```python
from build123d import *

# Parameters (mm, degrees)
F0_W     = 2
F0_H     = 50
F1_DEPTH = 45
F2_R     = 1.99999
F4_DEPTH = 40


# Not quite as in the source:
# - a fillet or chamfer is up to 0.001 mm smaller than in the source, because OpenCascade refuses the exact size


with BuildPart() as f1:
    # F0 (on Front) → F1 (new body)
    with BuildSketch(Plane.XZ):
        with Locations((-1, 25)):
            Rectangle(F0_W, F0_H)
    extrude(amount=F1_DEPTH)

    # F2 (radius 2 in the source; OpenCascade refuses exactly that, so slightly less here)
    f2_edges = [f1.edges().sort_by_distance(p)[0] for p in [
        (0, -22.5, 0),
        (0, -22.5, 50),
    ]]
    fillet(f2_edges, radius=F2_R)

    # F3 (on face) → F4 (cut)
    with BuildSketch(Plane.XZ.offset(45)):
        with BuildLine():
            Line((-2, 49.4142135624), (-2, 46.4142135624))
            ThreePointArc((-2, 46.4142135624), (-0.5, 47.9142135624), (-2, 49.4142135624))
        make_face()
        with BuildLine():
            ThreePointArc((-2, 0.5857864376), (-0.5056576806, 2.0857757678), (-2, 3.585765098))
            Line((-2, 3.585765098), (-2, 0.5857864376))
        make_face()
    extrude(amount=-F4_DEPTH, mode=Mode.SUBTRACT)


solid = f1.part
```
The listing builds one solid part. Answer for the finished solid, in the listing's coordinates (mm). A direction names the side the tool comes from. Round coordinates to 2 decimals unless told otherwise and drop trailing zeros. Order: outer loops, then holes, each group sorted by start corner. A loop starts at its lowest first (then second) coordinate and runs counter-clockwise, first axis right, second up. Notation, with made-up numbers: (64, 81) - (70, 81) arc R25 ccw to (70, 104) - close; hole circle Ø6 at (54.5, 68.5). An arc over 180 degrees is marked (long way). Put each result on its own line as item: value. Start each with the question number.
(1) Find section A-A (x = -1.2). Give the vertices of the cut face in (y, z), plus the area to 3 significant figures.
(2) Straight lines are drawn through the part: probe 1 along Z at (x, y) = (-1.75, -6.5); probe 2 along Z at (x, y) = (-0.95, -27); probe 3 along Z at (x, y) = (-0.2, -43). For each, find the intervals that lie inside material, in ascending order. Write a range as from..to.
(3) For faces 1 (the flat face through (-1, -5, 48)), 2 (the flat face through (-1, -45, 25)), determine the directions among +Z, -Z, +X, -X, +Y, -Y from which every point of the face is accessible in a straight line to the end or side of a thin tool.
(4) Given P1, Ø0.8, axis at x = -1.5, z = 48, coming from the -Y side; P2, Ø1, axis at x = -1, y = -30.5, coming from the -Z side, each flat-ended and moving along its own axis, determine where each tip first touches the part or whether it passes through.
(5) Determine the mould class of faces 3 (the cylindrical face through (-0.57, -22.82, 49.4)), 4 (the flat face through (-1, 0, 25)), 5 (the cylindrical face through (-0.506, -25.28, 2.053)) for opening direction Z: released by +Z, released by -Z, zero draft, split by the parting line, or undercut.
Reply:
1. outline: (-45, 0.17) - (0, 0.17) - (0, 49.83) - (-45, 49.83) - (-45, 49.18) - (-5, 49.18) - (-5, 46.65) - (-45, 46.65) - (-45, 3.35) - (-5, 3.35) - (-5, 0.82) - (-45, 0.82) - close
1. area: 2,030 mm^2
2. probe 1: 0.02..0.61, 3.56..46.44, 49.39..49.98
2. probe 2: 0.3..1.02, 3.15..46.84, 48.99..49.7
2. probe 3: 1.13..48.87
3. face 1: -X, -Y
3. face 2: +Z, -Z, +X, -X, -Y
4. P1: y = -5
4. P2: z = 0.06
5. face 3: released by +Z
5. face 4: zero draft
5. face 5: undercut
